Read the model definition and answer for the solid it produces. Units are mm, in the model's axes. Face numbers are marked on the shaded views. Give positions to 0.01 mm unless a question says otherwise; leave off trailing zeros. Order: outer loops, then holes, each group sorted by start corner. A loop starts at its lowest first (then second) coordinate and runs counter-clockwise, first axis right, second up.
Item 1: A cutting plane is placed at B-B (x = 0.5). Write down the section's boundary in (y, z).
Item 2: A cutting plane is placed at D-D (z = 62). Write down the section's boundary in (x, y).
Item 3: Given pin 1 Ø0.6 at (y, z) = (-185, 13) entering from +X; pin 2 Ø3.5 at (y, z) = (-181.5, -4) entering from -X; pin 3 Ø4.5 at (y, z) = (-74, 7) entering from +X; pin 4 Ø6.5 at (x, z) = (-13.5, 3) entering from +Y, each flat-ended and moving along its own axis, determine where each tip first touches the part or whether it passes through.
Item 4: Find the intervals of material crossed by line 1 along Z through (x, y) = (6.5, 111.5); line 2 along Z through (x, y) = (29.5, -202.5); line 3 along X through (y, z) = (-82, 1), in increasing order.
Item 5: A cutting plane is placed at A-A (y = -161). State how many separate pieces and enclosed holes the cut face has, plus the area to 3 significant figures.
Item 6: The mould has two halves that part along X. Classify the marked faces 1 and 2: +X half, -X half, draft (parallel to the pull), parting line (faces both ways), or undercut.
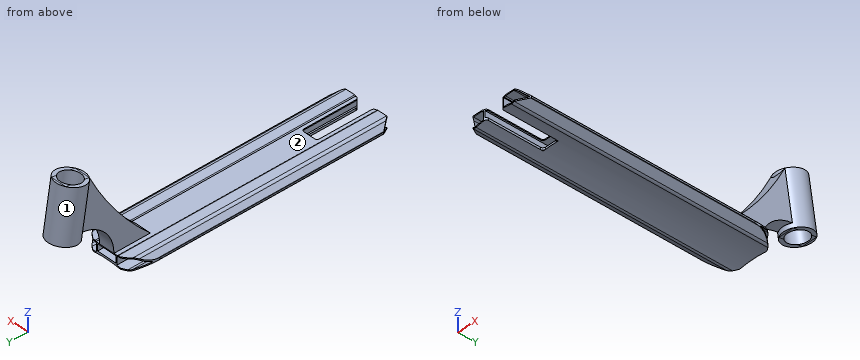
from build123d import *

# Parameters (mm, degrees)
F1_DEPTH       = 250
F2_W           = 38
F2_H           = 13
F3_DEPTH       = 500.001
F4_T1_DEPTH    = 509.3674969976
F5_R           = 9
F6_R           = 1
F8_DEPTH       = 500.001
F10_DEPTH      = 8.4253865001
F10_DEPTH_BACK = 15.0949186811
F12_DEPTH      = 15
F13_R          = 27.5
F14_DEPTH      = 100
F16_D          = 40
F18_DEPTH      = 8.4253866128
F18_DEPTH_BACK = 181.6948592657
F19_T1_DEPTH   = 2
F19_T6_DEPTH   = 16.7634824315
F19_S7_R       = 200
F19_T8_DEPTH   = 11
F19_T12_DEPTH  = 16.7634824315
F19_S13_R      = 200
F19_T14_DEPTH  = 11
F19_T15_DEPTH  = 27
F19_T17_DEPTH  = 29.2634824315


# Not quite as in the source:
# - a fillet or chamfer that OpenCascade refuses, or shapes differently, is made with other operations: its cross-section is extruded or revolved along the edge and cut away or added


with BuildPart() as f1:
    # F0 (on Front) → F1 (new body, symmetric)
    with BuildSketch(Plane.XZ):
        with BuildLine():
            Line((22.5, 13.7939186811), (0, 13.7939186811))
            Line((0, 13.7939186811), (-22.5, 13.7939186811))
            Line((-22.5, 13.7939186811), (-22.5, 15.0939186811))
            Line((-22.5, 15.0939186811), (-45.5824640741, 15.0939186811))
            Line((-45.5824640741, 15.0939186811), (-57.5, 5.0939186811))
            Line((-57.5, 5.0939186811), (-57.5, 1.0939186811))
            Line((-57.5, 1.0939186811), (-40.1794919243, -8.9060813189))
            ThreePointArc((-40.1794919243, -8.9060813189), (0, -4.8285364604), (40.1794919243, -8.9060813189))
            Line((40.1794919243, -8.9060813189), (57.5, 1.0939186811))
            Line((57.5, 1.0939186811), (57.5, 5.0939186811))
            Line((57.5, 5.0939186811), (45.5824640741, 15.0939186811))
            Line((45.5824640741, 15.0939186811), (22.5, 15.0939186811))
            Line((22.5, 15.0939186811), (22.5, 13.7939186811))
        make_face()
    extrude(amount=F1_DEPTH, both=True)

    # F2 (on face) → F3 (cut, through all)
    with BuildSketch(Plane.XZ.offset(250)):
        with Locations((0, 5.2939186811)):
            Rectangle(F2_W, F2_H)
    extrude(amount=-F3_DEPTH, mode=Mode.SUBTRACT)

    # F4: fillet of radius 2 on 2 edges, made by hand

    # F4_s2 → F4_t1 (cut)
    with BuildSketch(Plane.XZ.offset(-254.6837484988)):
        with BuildLine():
            ThreePointArc((24.3734993995, 15.0939186811), (23.2333239744, 14.7370863537), (22.5, 13.7939186811))
            Line((22.5, 13.7939186811), (22.5, 15.0939186811))
            Line((22.5, 15.0939186811), (24.3734993995, 15.0939186811))
        make_face()
        with BuildLine():
            ThreePointArc((-24.3734993995, 15.0939186811), (-23.2333239744, 14.7370863537), (-22.5, 13.7939186811))
            Line((-22.5, 13.7939186811), (-22.5, 15.0939186811))
            Line((-22.5, 15.0939186811), (-24.3734993995, 15.0939186811))
        make_face()
    extrude(amount=F4_T1_DEPTH, mode=Mode.SUBTRACT)

    # F5
    f5_edges = [f1.edges().sort_by_distance(p)[0] for p in [
        (45.582464, 0, 15.093919),
        (-45.582464, 0, 15.093919),
        (-40.179492, 0, -8.906081),
        (40.179492, 0, -8.906081),
    ]]
    fillet(f5_edges, radius=F5_R)

    # F6
    f6_edges = [f1.edges().sort_by_distance(p)[0] for p in [
        (57.5, 0, 1.093919),
        (57.5, 0, 5.093919),
        (-57.5, 0, 5.093919),
        (-57.5, 0, 1.093919),
    ]]
    fillet(f6_edges, radius=F6_R)

    # F7 (on face) → F8 (cut, through all)
    with BuildSketch(Plane.XZ.offset(250)):
        with BuildLine():
            Line((-55.6135241478, 2.3141624168), (-42.1022690923, -5.4865643266))
            ThreePointArc((-42.1022690923, -5.4865643266), (-39.7790673433, -6.3247593796), (-37.3093701274, -6.3039513313))
            ThreePointArc((-37.3093701274, -6.3039513313), (-29.1789785809, -4.9471035834), (-21, -3.9230860615))
            Line((-21, -3.9230860615), (-21, 11.7939186811))
            Line((-21, 11.7939186811), (-22.6125713953, 11.7939186811))
            ThreePointArc((-22.6125713953, 11.7939186811), (-23.3458953697, 12.7370863537), (-24.4860707948, 13.0939186811))
            Line((-24.4860707948, 13.0939186811), (-42.3067319657, 13.0939186811))
            ThreePointArc((-42.3067319657, 13.0939186811), (-44.7008729689, 12.6717670266), (-46.8062452335, 11.456229783))
            Line((-46.8062452335, 11.456229783), (-55.7563117574, 3.9462322637))
            ThreePointArc((-55.7563117574, 3.9462322637), (-56.1097188459, 3.0930320778), (-55.6135241478, 2.3141624168))
        make_face()
        with BuildLine():
            ThreePointArc((21, -3.9230860615), (29.1789785809, -4.9471035834), (37.3093701274, -6.3039513313))
            ThreePointArc((37.3093701274, -6.3039513313), (39.7790673433, -6.3247593796), (42.1022690923, -5.4865643266))
            Line((42.1022690923, -5.4865643266), (55.6135241478, 2.3141624168))
            ThreePointArc((55.6135241478, 2.3141624168), (56.1097188459, 3.0930320778), (55.7563117574, 3.9462322637))
            Line((55.7563117574, 3.9462322637), (46.8062452335, 11.456229783))
            ThreePointArc((46.8062452335, 11.456229783), (44.7008729689, 12.6717670266), (42.3067319657, 13.0939186811))
            Line((42.3067319657, 13.0939186811), (24.4860707948, 13.0939186811))
            ThreePointArc((24.4860707948, 13.0939186811), (23.3458953697, 12.7370863537), (22.6125713953, 11.7939186811))
            Line((22.6125713953, 11.7939186811), (21, 11.7939186811))
            Line((21, 11.7939186811), (21, -3.9230860615))
        make_face()
    extrude(amount=-F8_DEPTH, mode=Mode.SUBTRACT)

    # F9 (on Top) → F10 (cut, two sides)
    with BuildSketch(Plane.XY) as f10_sk:
        with BuildLine():
            ThreePointArc((-57.5, 200), (0, 257.5), (57.5, 200))
            Line((57.5, 200), (57.5, 280))
            Line((57.5, 280), (-57.5, 280))
            Line((-57.5, 280), (-57.5, 200))
        make_face()
    extrude(amount=-F10_DEPTH, mode=Mode.SUBTRACT)
    extrude(f10_sk.sketch, amount=F10_DEPTH_BACK, mode=Mode.SUBTRACT)

    # F11 (on Right) → F12 (join, symmetric)
    with BuildSketch(Plane.YZ):
        with BuildLine():
            ThreePointArc((297.3819995028, 173.7939186811), (245.9666940414, 88.4561965341), (180, 13.7939186811))
            Line((180, 13.7939186811), (250, 13.7939186811))
            ThreePointArc((250, 13.7939186811), (267.6550746197, 60.2698133678), (311.7145367693, 83.3018398057))
            Line((311.7145367693, 83.3018398057), (313.0254460068, 75.0250846216))
            Line((313.0254460068, 75.0250846216), (358.4591096742, 82.2210700135))
            Line((358.4591096742, 82.2210700135), (342.8156631702, 180.989904073))
            Line((342.8156631702, 180.989904073), (297.3819995028, 173.7939186811))
        make_face()
    extrude(amount=F12_DEPTH, both=True)

    # F13 (on face) → F14 (join, through all)
    with BuildSketch(Plane(origin=(0, -19.5751816724, 123.5928329339), x_dir=(1, 0, 0), z_dir=(0, -0.156434465, 0.9876883406))):
        with Locations((0, 343.9080923079)):
            Circle(F13_R)
    extrude(amount=-F14_DEPTH)

    # F16 (through all)
    with Locations(Plane(origin=(0, -19.5751816724, 123.5928329339), x_dir=(1, 0, 0), z_dir=(0, -0.156434465, 0.9876883406))):
        with Locations((0, 343.9080923079)):
            Hole(F16_D / 2)

    # F17 (on Top) → F18 (cut, two sides)
    with BuildSketch(Plane.XY) as f18_sk:
        Polygon((-43.2975540478, -250), (-68, -216), (-68, -346), (68, -346), (68, -216), (43.2975540478, -250), (16, -250), (16, -140), (-16, -140), (-16, -250), align=None)
    extrude(amount=-F18_DEPTH, mode=Mode.SUBTRACT)
    extrude(f18_sk.sketch, amount=F18_DEPTH_BACK, mode=Mode.SUBTRACT)

    # F19: fillet of radius 5 on 8 edges, made by hand

    # F19_s2 → F19_t1 (join)
    with BuildSketch(Plane.XY.offset(11.7939186811)):
        with BuildLine():
            ThreePointArc((-11, -140), (-14.5355339059, -141.4644660941), (-16, -145))
            Line((-16, -145), (-16, -140))
            Line((-16, -140), (-11, -140))
        make_face()
        with BuildLine():
            ThreePointArc((16, -145), (14.5355339059, -141.4644660941), (11, -140))
            Line((11, -140), (16, -140))
            Line((16, -140), (16, -145))
        make_face()
    extrude(amount=F19_T1_DEPTH)


with BuildPart() as f19_tool4:
    # F19_s5 → F19_t6 (new body)
    with BuildSketch(Plane.XY.offset(-1.2060813189)):
        with BuildLine():
            ThreePointArc((-16, -145), (-14.5355339059, -141.4644660941), (-11, -140))
            Line((-11, -140), (-16, -140))
            Line((-16, -140), (-16, -145))
        make_face()
    extrude(amount=-F19_T6_DEPTH)

    # F19_s7 → F19_t8 (cut, symmetric)
    with BuildSketch(Plane.XZ.offset(142.5)):
        with Locations((0, -204.8285364604)):
            Circle(F19_S7_R)
    extrude(amount=F19_T8_DEPTH, both=True, mode=Mode.SUBTRACT)


with BuildPart() as f1_1:
    add(f1.part)

    # F19_t3: union F19_tool4
    add(f19_tool4.part)


with BuildPart() as f19_tool10:
    # F19_s11 → F19_t12 (new body)
    with BuildSketch(Plane.XY.offset(-17.9695637504)):
        with BuildLine():
            ThreePointArc((11, -140), (14.5355339059, -141.4644660941), (16, -145))
            Line((16, -145), (16, -140))
            Line((16, -140), (11, -140))
        make_face()
    extrude(amount=F19_T12_DEPTH)

    # F19_s13 → F19_t14 (cut, symmetric)
    with BuildSketch(Plane.XZ.offset(142.5)):
        with Locations((0, -204.8285364604)):
            Circle(F19_S13_R)
    extrude(amount=F19_T14_DEPTH, both=True, mode=Mode.SUBTRACT)


with BuildPart() as f1_2:
    add(f1_1.part)

    # F19_t9: union F19_tool10
    add(f19_tool10.part)

    # F19_s16 → F19_t15 (cut)
    with BuildSketch(Plane.XY.offset(-0.7060813189)):
        with BuildLine():
            ThreePointArc((-21, -250), (-17.4644660941, -248.5355339059), (-16, -245))
            Line((-16, -245), (-16, -250))
            Line((-16, -250), (-21, -250))
        make_face()
        with BuildLine():
            ThreePointArc((21, -250), (17.4644660941, -248.5355339059), (16, -245))
            Line((16, -245), (16, -250))
            Line((16, -250), (21, -250))
        make_face()
    extrude(amount=F19_T15_DEPTH, mode=Mode.SUBTRACT)

    # F19_s18 → F19_t17 (cut)
    with BuildSketch(Plane.XY.offset(-17.9695637504)):
        with BuildLine():
            ThreePointArc((21, -250), (17.4644660941, -248.5355339059), (16, -245))
            Line((16, -245), (16, -250))
            Line((16, -250), (21, -250))
        make_face()
        with BuildLine():
            ThreePointArc((-21, -250), (-17.4644660941, -248.5355339059), (-16, -245))
            Line((-16, -245), (-16, -250))
            Line((-16, -250), (-21, -250))
        make_face()
    extrude(amount=F19_T17_DEPTH, mode=Mode.SUBTRACT)


solid = f1_2.part
Response values:
1. outline: (-140, -4.83) - (250, -4.83) - (250, -1.21) - (-140, -1.21) - close; (-140, 11.79) - (250, 11.79) - (250, 13.79) arc R70 cw to (307.27, 82.63) - (308.59, 74.32) - (315.99, 75.5) - (300.35, 174.26) - (292.94, 173.09) - (293.94, 166.81) arc R550 cw to (180, 13.79) - (-140, 13.79) - close; (339.85, 180.52) - (355.49, 81.75) - (362.9, 82.92) - (347.26, 181.69) - close
2. outline: (-15, 225.29) - (15, 225.29) - (15, 269.24) - (-15, 269.24) - close
3. pin 1: stops at x = 48.44
3. pin 2: stops at x = -51.71
3. pin 3: stops at x = 57.49
3. pin 4: passes through
4. line 1: z = -4.93 to -1.21, 11.79 to 13.79
4. line 2: z = -7.02 to -4.99, 13.09 to 15.09
4. line 3: x = -57.24 to -53.34, -21 to -19, 19 to 21, 53.34 to 57.24
5. separate pieces: 2
5. enclosed holes: 2
5. area: 434 mm2
6. face 1: parting line
6. face 2: undercut
